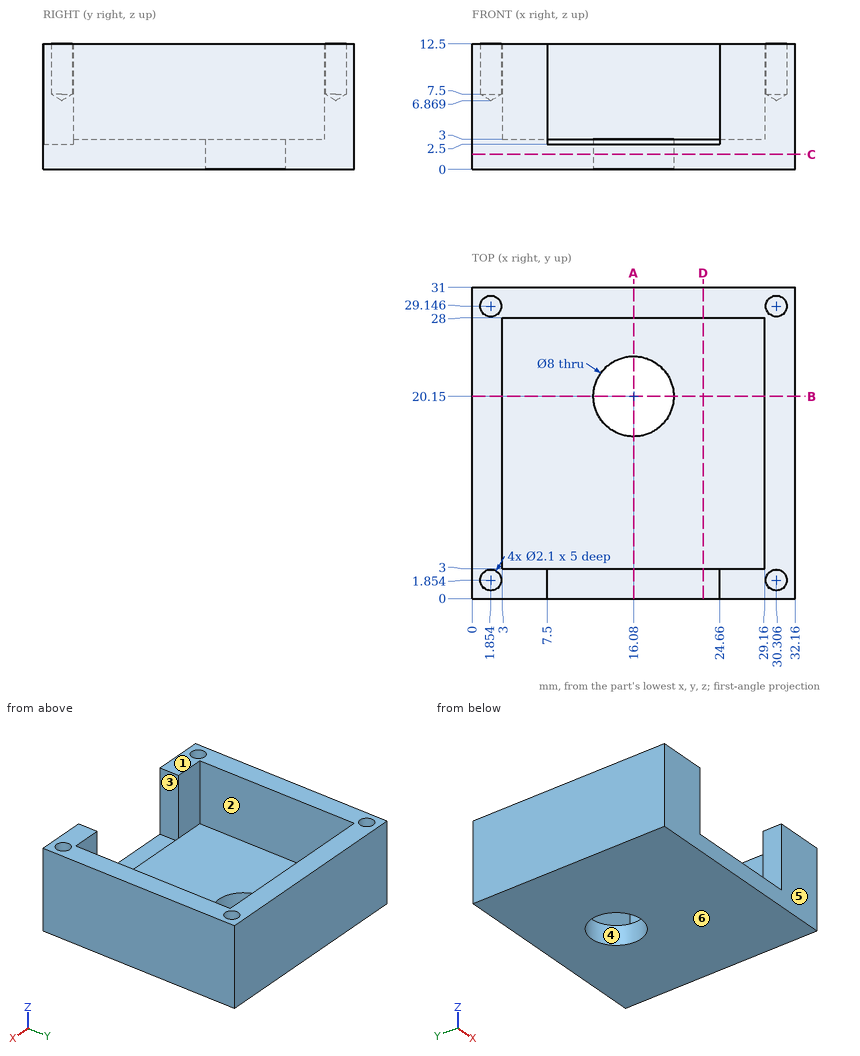
Geometry: see drawing. Coordinates: mm, zero at the bounding-box minimum. A direction names the side the tool comes from. Round coordinates to 2 decimals unless told otherwise and drop trailing zeros. Order: outer loops, then holes, each group sorted by start corner. A loop starts at its lowest first (then second) coordinate and runs counter-clockwise, first axis right, second up. Notation, with made-up numbers: (-26.75, -16) -> (17.25, -16) arc R31 ccw to (17.25, 18) -> close; hole circle Ø11 at (-18.75, 25). An arc over 180 degrees is marked (long way). Write each question's results on one line, items separated by ' | '.
Q1. Pull-direction query (Y, two-part tool) for the marked faces 4, 5 and 6; classes: released by +Y, released by -Y, zero draft, split by the parting line, or undercut.
Response values:
face 4: undercut | face 5: released by -Y | face 6: zero draft
Q2. Section query B-B (y = 20.15). Output: boundary loops of the cut face in (x, z).
Response values:
outline: (0, 0) -> (12.08, 0) -> (12.08, 3) -> (3, 3) -> (3, 12.5) -> (0, 12.5) -> close; (20.08, 0) -> (32.16, 0) -> (32.16, 12.5) -> (29.16, 12.5) -> (29.16, 3) -> (20.08, 3) -> close
Q3. Ray query, line 1 along X through (y, z) = (24.5, 11); line 2 along Y through (x, z) = (23.5, 5.5); line 3 along Z through (x, y) = (27.5, 22.5). Return the intervals inside material, ascending.
Response values:
line 1: 0 to 3, 29.16 to 32.16 | line 2: 28 to 31 | line 3: 0 to 3
Q4. Section query A-A (x = 16.08). Output: boundary loops of the cut face in (y, z).
Response values:
outline: (0, 0) -> (16.15, 0) -> (16.15, 3) -> (3, 3) -> (3, 2.5) -> (0, 2.5) -> close; (24.15, 0) -> (31, 0) -> (31, 12.5) -> (28, 12.5) -> (28, 3) -> (24.15, 3) -> close
Q5. Section query D-D (x = 23). Output: boundary loops of the cut face in (y, z), and give its area (3 significant figures).
Response values:
outline: (0, 0) -> (31, 0) -> (31, 12.5) -> (28, 12.5) -> (28, 3) -> (3, 3) -> (3, 2.5) -> (0, 2.5) -> close | area: 120 mm²
Q6. Pin query (flat end, axial travel): pin 1 Ø1.9 at (x, y) = (30.31, 1.85) entering from +Z (1 decimal); pin 2 Ø1.5 at (x, z) = (12.5, 8.5) entering from -Y; pin 3 Ø5 at (x, y) = (16.08, 20.15) entering from +Z; pin 4 Ø8 at (x, y) = (7.5, 19.5) entering from +Z. Return the tip coordinate at first contact, or that it passes through.
Response values:
pin 1: z = 7.4 | pin 2: y = 28 | pin 3: through | pin 4: z = 3
Q7. Section query C-C (z = 1.5). Output: boundary loops of the cut face in (x, y), and give its area (3 significant figures).
Response values:
outline: (0, 0) -> (32.16, 0) -> (32.16, 31) -> (0, 31) -> close; hole circle Ø8 at (16.08, 20.15) | area: 947 mm²
Q8. Access query for the marked faces 1, 2 and 3. Directions: +Z, -Z, +X, -X, +Y, -Y. A direction counts if a zero-diameter tool reaches every point of the face in a straight line with its end or side. Return the directions, or none.
Response values:
face 1: +Z, +X, -X, +Y, -Y | face 2: +Z | face 3: +Z, -Y
